from build123d import *

# Parameters (mm, degrees)
BOX3529_W        = 1400
BOX3529_H        = 850
BOX3529_DEPTH    = 500
ARRAY281_Z_COUNT = 4
ARRAY281_Z_PITCH = 550
BOX3527_W        = 500
BOX3527_H        = 400
BOX3527_DEPTH    = 2200
BOX3528_W        = 1500
BOX3528_H        = 500
BOX3528_DEPTH    = 2200


with BuildPart() as array281:
    # Box3529 → Box3529 (new body)
    with BuildSketch(Plane(origin=(1550, -300, 0), x_dir=(1, 0, 0), z_dir=(0, 0, 1))):
        with Locations((700, 425)):
            Rectangle(BOX3529_W, BOX3529_H)
    extrude(amount=BOX3529_DEPTH)

    # Array281 Z: Array281 ×4


with BuildPart() as array281_1:
    add(array281.part)
    with Locations(*[(0, 0, i * ARRAY281_Z_PITCH) for i in range(1, ARRAY281_Z_COUNT)]):
        add(array281.part)


with BuildPart() as box3527:
    # Box3527 → Box3527 (new body)
    with BuildSketch(Plane(origin=(2500, 200, 0), x_dir=(1, 0, 0), z_dir=(0, 0, 1))):
        with Locations((250, 200)):
            Rectangle(BOX3527_W, BOX3527_H)
    extrude(amount=BOX3527_DEPTH)


with BuildPart() as cut003:
    # Box3528 → Box3528 (new body)
    with BuildSketch(Plane(origin=(1500, -300, 0), x_dir=(1, 0, 0), z_dir=(0, 0, 1))):
        with Locations((750, 250)):
            Rectangle(BOX3528_W, BOX3528_H)
    extrude(amount=BOX3528_DEPTH)

    # Fusion015: union Box3527
    add(box3527.part)

    # Cut003: cut Array281
    add(array281_1.part, mode=Mode.SUBTRACT)


solid = cut003.part
Geometry: final body of the model. Coordinates: model frame, mm. A direction names the side the tool comes from. Round coordinates to 2 decimals unless told otherwise and drop trailing zeros. Write each loop counter-clockwise with the first axis right and the second up, starting at its lowest first coordinate (ties: lowest second). Pieces come first, ordered by that corner, then holes. Notation, with made-up numbers: M 43.5,-20 L 101.5,-20 A17 cw 101.5,-6 Z; hole C -12,76.25 d10. An arc over 180 degrees is marked long. Write item = value, one per line.
Item 1: Access query for faces 1 (the face through (2950, 119, 796)), 2 (the face through (2950, 119, 246)), 3 (the face through (1550, -53, 1346)), 4 (the face through (1850, 200, 1095)), 5 (the face through (2722, 550, 246)). Directions: +Z, -Z, +X, -X, +Y, -Y. A direction counts if a zero-diameter tool reaches every point of the face in a straight line with its end or side. Return the directions, or none.
Findings:
face_1 = -Y
face_2 = -Z, -Y
face_3 = +Y, -Y
face_4 = +Z, -Z, -X, +Y
face_5 = -Z, -X, -Y
Item 2: Section query C-C on y = -198. Return loops of the section in (x, z), then the cut area to 3 significant figures.
Findings:
outline = M 1500,0 L 1550,0 L 1550,500 L 2950,500 L 2950,0 L 3000,0 L 3000,2200 L 1500,2200 Z; hole M 1550,550 L 2950,550 L 2950,1050 L 1550,1050 Z; hole M 1550,1100 L 2950,1100 L 2950,1600 L 1550,1600 Z; hole M 1550,1650 L 2950,1650 L 2950,2150 L 1550,2150 Z
area = 500,000 mm^2
Item 3: Section query B-B on z = 901. Return loops of the section in (x, y), then the cut area to 3 significant figures.
Findings:
outline = M 1500,-300 L 1550,-300 L 1550,200 L 1500,200 Z; M 2500,550 L 2950,550 L 2950,-300 L 3000,-300 L 3000,600 L 2500,600 Z
area = 92,500 mm^2
Item 4: Pin query (flat end, axial travel): P1, Ø5, axis at x = 1785.5, y = 191, coming from the -Z side; P2, Ø5, axis at y = 426.5, z = 1905.5, coming from the -X side. Return the tip coordinate at first contact, or that it passes through.
Findings:
P1 = 500
P2 = 2950
Item 5: Pull-direction query (Z, two-part tool) for faces 6 (the face through (2396, 37, 550)), 7 (the face through (1550, -53, 246)), 8 (the face through (2953, 319, 0)), 9 (the face through (1550, -53, 796)); classes: pulls with the +Z half, pulls with the -Z half, needs draft (parallel to the pull), parting line crosses it, or undercut.
Findings:
face_6 = undercut
face_7 = needs draft
face_8 = pulls with the -Z half
face_9 = undercut
Item 6: Material intervals for line 1 along Z through (x, y) = (1804, -31); line 2 along X through (y, z) = (156, 642.5); line 3 along Y through (x, z) = (2599, 1651.5), sorted ascending. Write a range as [from, to].
Findings:
line_1 = [500, 550], [1050, 1100], [1600, 1650], [2150, 2200]
line_2 = [1500, 1550], [2950, 3000]
line_3 = [550, 600]
Item 7: Section query A-A on x = 2234. Return loops of the section in (y, z), then the cut area to 3 significant figures.
Findings:
outline = M -300,500 L 200,500 L 200,550 L -300,550 Z; M -300,1050 L 200,1050 L 200,1100 L -300,1100 Z; M -300,1600 L 200,1600 L 200,1650 L -300,1650 Z; M -300,2150 L 200,2150 L 200,2200 L -300,2200 Z
area = 100,000 mm^2
Item 8: Section query D-D on y = 439.5. Return loops of the section in (x, z), then the cut area to 3 significant figures.
Findings:
outline = M 2500,500 L 2950,500 L 2950,0 L 3000,0 L 3000,2200 L 2500,2200 L 2500,2150 L 2950,2150 L 2950,1650 L 2500,1650 L 2500,1600 L 2950,1600 L 2950,1100 L 2500,1100 L 2500,1050 L 2950,1050 L 2950,550 L 2500,550 Z
area = 200,000 mm^2
